Here's how the part is built. I have some questions about the finished solid (model axes, mm). A direction names the side the tool comes from. Round coordinates to 2 decimals unless told otherwise and drop trailing zeros. Loops run counter-clockwise (first coordinate to the right, second up) from the corner with the lowest first, then second, coordinate; pieces in that order, holes last. Notation, with made-up numbers: (50, 60) -> (99, 60) arc R25 ccw to (99, 99) -> close; hole circle Ø9 at (77, -11). An arc over 180 degrees is marked (long way). Use CSV: the item, a comma, the result in double quotes. Start each with the question number.
from build123d import *

# Parameters (mm, degrees)
F0_W     = 180
F0_H     = 40
F1_DEPTH = 40
F2_T     = -2


with BuildPart() as f1:
    # F0 (on Right) → F1 (new body, symmetric)
    with BuildSketch(Plane.YZ):
        with Locations((9.012016, -23.53282)):
            Rectangle(F0_W, F0_H)
    extrude(amount=F1_DEPTH, both=True)

    # F2
    f2_openings = [f1.faces().sort_by_distance(p)[0] for p in [
        (0, 9.012016, -3.53282),
        (0, 9.012016, -43.53282),
    ]]
    offset(amount=F2_T, openings=f2_openings)


solid = f1.part
Q1. I want a section at A-A, the plane y = -41.5. List the corners of the cut face in (x, z) for me, then the cut area to 3 significant figures.
Q2. I want a section at C-C, the plane z = -12. List the corners of the cut face in (x, y) for me.
Q3. If we mould it in two halves opening along X, with no side actions, what happens to faces 3 (the flat face through (-40, 8, -23)), 4 (the flat face through (39, 9, -3.533)), 5 (the flat face through (1, 97.012, -24))? For each: pulls with the +X half, pulls with the -X half, needs draft (parallel to the pull), parting line crosses it, or undercut.
Q4. I want a section at B-B, the plane x = -8.5. List the corners of the cut face in (y, z) for me.
Q5. I need wall thicknesses on line 1 along Y through (x, z) = (-35.5, -9); line 2 along X through (y, z) = (29.5, -26). Which ranges of each line are inside material? Lowest first, please.
Q6. For faces 1 (the flat face through (1, -78.988, -24)), 2 (the flat face through (39, 9, -43.533)), which set-ups out of +Z, -Z, +X, -X, +Y, -Y let a thin tool reach every point of the face, with its end or its side?
Values found:
1,outline,"(-40, -43.53) -> (-38, -43.53) -> (-38, -3.53) -> (-40, -3.53) -> close; (38, -43.53) -> (40, -43.53) -> (40, -3.53) -> (38, -3.53) -> close"
1,area,"160 mm2"
2,outline,"(-40, -80.99) -> (40, -80.99) -> (40, 99.01) -> (-40, 99.01) -> close; hole (-38, -78.99) -> (38, -78.99) -> (38, 97.01) -> (-38, 97.01) -> close"
3,face 3,"pulls with the -X half"
3,face 4,"needs draft"
3,face 5,"undercut"
4,outline,"(-80.99, -43.53) -> (-78.99, -43.53) -> (-78.99, -3.53) -> (-80.99, -3.53) -> close; (97.01, -43.53) -> (99.01, -43.53) -> (99.01, -3.53) -> (97.01, -3.53) -> close"
5,line 1,"-80.99 to -78.99, 97.01 to 99.01"
5,line 2,"-40 to -38, 38 to 40"
6,face 1,"+Z, -Z"
6,face 2,"-Z, +X, -X, +Y, -Y"
